```python
from build123d import *

# Parameters (mm, degrees)
SKETCH1_R           = 9.525
BOSS_EXTRUDE1_DEPTH = 20.985
CHAMFER1_SIZE       = 0.5


with BuildPart() as part:
    # Sketch1 → Boss-Extrude1 (new body)
    with BuildSketch(Plane(origin=(0, 0, 0), x_dir=(1, 0, 0), z_dir=(0, 1, 0))):
        with BuildLine():
            ThreePointArc((-9.662407992, 18.498593241), (0, 11.075), (9.662407992, 18.498593241))
            ThreePointArc((9.662407992, 18.498593241), (9.784456714, 18.715644618), (9.996061597, 18.846909862))
            ThreePointArc((9.996061597, 18.846909862), (35.65, 0), (9.996061597, -18.846909862))
            ThreePointArc((9.996061597, -18.846909862), (9.784456714, -18.715644618), (9.662407992, -18.498593241))
            ThreePointArc((9.662407992, -18.498593241), (0, -11.075), (-9.662407992, -18.498593241))
            ThreePointArc((-9.662407992, -18.498593241), (-9.784456714, -18.715644618), (-9.996061597, -18.846909862))
            ThreePointArc((-9.996061597, -18.846909862), (-35.65, 0), (-9.996061597, 18.846909862))
            ThreePointArc((-9.996061597, 18.846909862), (-9.784456714, 18.715644618), (-9.662407992, 18.498593241))
        make_face()
        with Locations(Location((-15.9, 0, 0), (0, 0, 270))):
            Circle(SKETCH1_R, mode=Mode.SUBTRACT)
        with Locations(Location((15.9, 0, 0), (0, 0, 270))):
            Circle(SKETCH1_R, mode=Mode.SUBTRACT)
    extrude(amount=BOSS_EXTRUDE1_DEPTH)

    # Chamfer1
    chamfer1_edges = [part.edges().sort_by_distance(p)[0] for p in [
        (-15.9, 0, -9.525),
        (-15.9, 20.985, -9.525),
        (15.9, 0, -9.525),
        (15.9, 20.985, -9.525),
    ]]
    chamfer(chamfer1_edges, length=CHAMFER1_SIZE)


solid = part.part
```
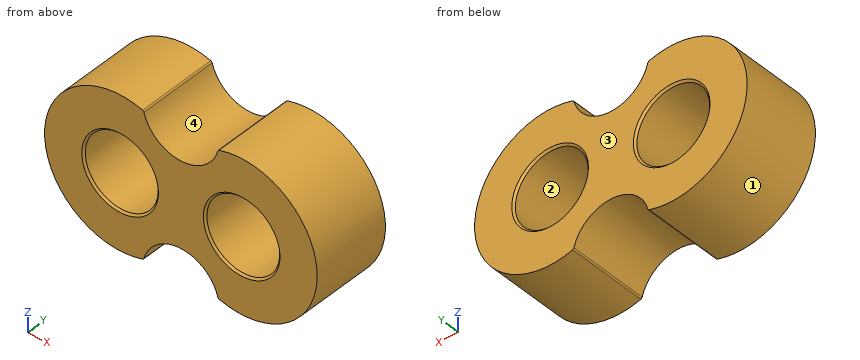
For this review, take the finished solid that the model builds, in its own axes (mm). Face numbers are marked on the shaded views. Coordinates: 2 decimals unless noted, no trailing zeros. Loops run counter-clockwise (first coordinate to the right, second up) from the corner with the lowest first, then second, coordinate; pieces in that order, holes last. Notation, with made-up numbers: (29.25, 32.5) - (85.25, 32.5) arc R22 cw to (85.25, 64.5) - close; hole circle Ø6 at (81, -20). An arc over 180 degrees is marked (long way). Use one line per item in the form item = value. Start each with the question number.
1) For pin 1 (1.5 mm diameter, centred on y = 10.5, z = 4.5, fed in from -X); pin 2 (1 mm diameter, centred on x = -6.5, y = 2, fed in from -Z); pin 3 (1 mm diameter, centred on y = 11, z = -7, fed in from -X); pin 4 (1 mm diameter, centred on x = -15, z = -8.5, fed in from +Y), all flat-tipped, find the tip position at first contact; note any pin that passes through.
2) Take a section at B-B (x = -15.9). State the section outline as (y, z) points (3 decimals).
3) Take a section at D-D (z = 12). State the section outline as (x, y) points (3 decimals), plus the area to 3 significant figures.
4) To check wall thickness, follow probe 1 along X at (y, z) = (15.25, 0) (3 decimals); probe 2 along X at (y, z) = (6, -2.5); probe 3 along X at (y, z) = (18.5, 17). State the ranges of each line that lie inside material, in increasing order. Write a range as from..to.
5) Take a section at A-A (z = 0). State the section outline as (x, y) points (3 decimals), plus the area to 3 significant figures.
6) Take a section at C-C (y = 6.5). State the section outline as (x, z) points (3 decimals).
7) Draft analysis for pull direction Z (two halves, no side actions). For the marked faces 1, 2, 3 and 4, state which applies: released by +Z, released by -Z, zero draft, split by the parting line, or undercut.
From the geometry:
q1.pin_1 = -35.29
q1.pin_2 = -13.93
q1.pin_3 = -34.55
q1.pin_4 = through
q2.outline = (0, -19.75) - (20.985, -19.75) - (20.985, -10.025) - (20.485, -9.525) - (0.5, -9.525) - (0, -10.025) - close; (0, 10.025) - (0.5, 9.525) - (20.485, 9.525) - (20.985, 10.025) - (20.985, 19.75) - (0, 19.75) - close
q3.outline = (-31.586, 0) - (-4.201, 0) - (-4.201, 20.985) - (-31.586, 20.985) - close; (4.201, 0) - (31.586, 0) - (31.586, 20.985) - (4.201, 20.985) - close
q3.area = 1,150 mm2
q4.probe_1 = -35.65..-25.425, -6.375..6.375, 25.425..35.65
q4.probe_2 = -35.49..-25.09, -6.71..6.71, 25.09..35.49
q4.probe_3 = -25.95..-9.13, 9.13..25.95
q5.outline = (-35.65, 0) - (-25.925, 0) - (-25.425, 0.5) - (-25.425, 20.485) - (-25.925, 20.985) - (-35.65, 20.985) - close; (-6.375, 0.5) - (-5.875, 0) - (5.875, 0) - (6.375, 0.5) - (6.375, 20.485) - (5.875, 20.985) - (-5.875, 20.985) - (-6.375, 20.485) - close; (25.425, 0.5) - (25.925, 0) - (35.65, 0) - (35.65, 20.985) - (25.925, 20.985) - (25.425, 20.485) - close
q5.area = 696 mm2
q6.outline = (-9.996, -18.847) arc R0.5 ccw to (-9.662, -18.499) arc R10 cw to (9.662, -18.499) arc R0.5 ccw to (9.996, -18.847) arc R19.75 ccw (long way) to (9.996, 18.847) arc R0.5 ccw to (9.662, 18.499) arc R10 cw to (-9.662, 18.499) arc R0.5 ccw to (-9.996, 18.847) arc R19.75 ccw (long way) to start; hole circle Ø19.05 at (-15.9, 0); hole circle Ø19.05 at (15.9, 0)
q7.face_1 = split by the parting line
q7.face_2 = undercut
q7.face_3 = zero draft
q7.face_4 = released by +Z
